Can you work these out from the drawing? Everything is in mm from the part's minimum corner. Give positions to 0.01 mm unless a question says otherwise; leave off trailing zeros. Order: outer loops, then holes, each group sorted by start corner. A loop starts at its lowest first (then second) coordinate and runs counter-clockwise, first axis right, second up. Notation, with made-up numbers: (9.25, 17.25) - (26.25, 17.25) arc R22 ccw to (26.25, 29.25) - close; hole circle Ø11 at (64.25, -18). An arc over 180 degrees is marked (long way). Answer as a JSON object with one key per item and string values.
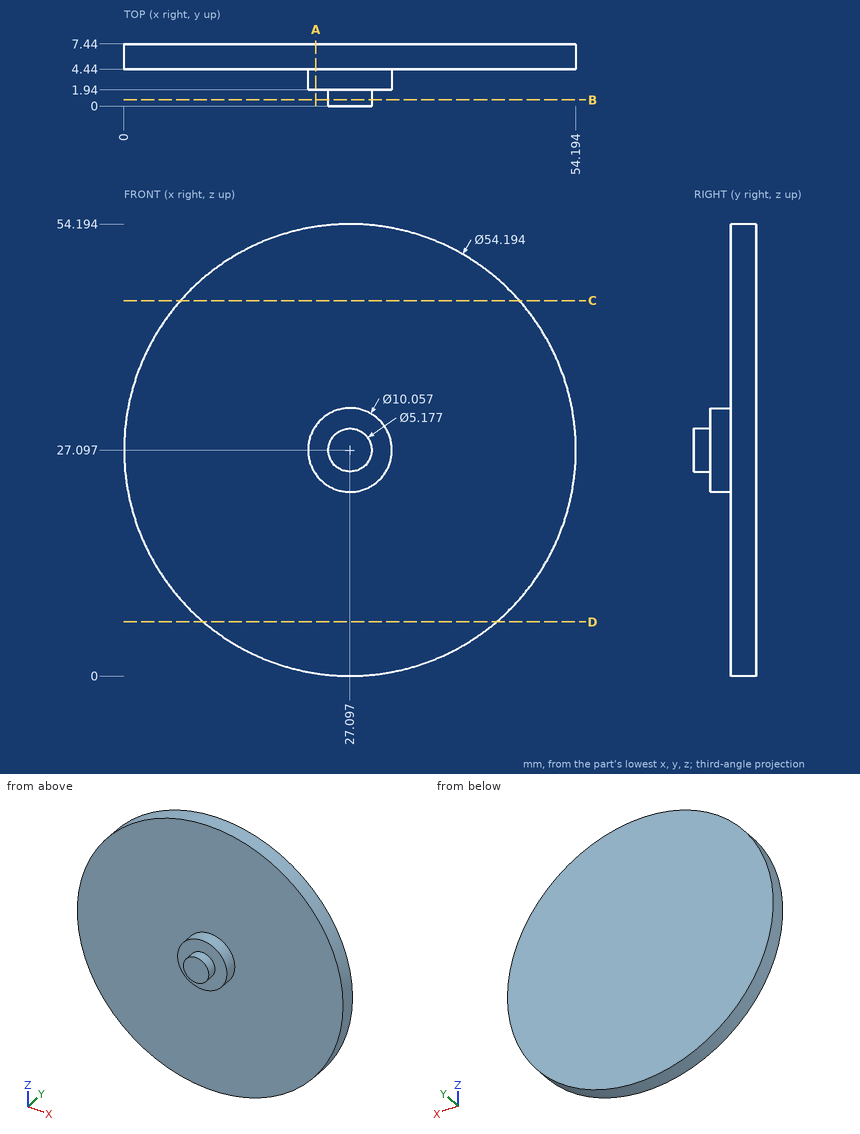
Q1. If we section it at B-B, the plane y = 0.75: Please give me the cut outline in (x, z) (1 decimal).
Recorded:
{"outline": "circle Ø5.2 at (27.1, 27.1)"}
Q2. If we section it at A-A, the plane x = 23: Please give me the cut outline in (y, z).
Recorded:
{"outline": "(1.94, 24.18) - (4.44, 24.18) - (4.44, 0.31) - (7.44, 0.31) - (7.44, 53.88) - (4.44, 53.88) - (4.44, 30.01) - (1.94, 30.01) - close"}
Q3. If we section it at D-D, the plane z = 6.5: Please give me the cut outline in (x, y), then the cut area to 3 significant figures.
Recorded:
{"outline": "(9.49, 4.44) - (44.7, 4.44) - (44.7, 7.44) - (9.49, 7.44) - close", "area": "106 mm^2"}
Q4. If we section it at C-C, the plane z = 45: Please give me the cut outline in (x, y).
Recorded:
{"outline": "(6.76, 4.44) - (47.44, 4.44) - (47.44, 7.44) - (6.76, 7.44) - close"}
Q5. I'm going to push flat-ended pins straight in: pin 1 Ø3 at (x, z) = (26.5, 24.5) entering from -Y; pin 2 Ø1.5 at (y, z) = (4.5, 33.5) entering from -X; pin 3 Ø1.5 at (y, z) = (4.5, 47) entering from -X; pin 4 Ø1.5 at (y, z) = (4, 30) entering from -X. Where does each tip first touch, or does it pass through?
Recorded:
{"pin 1": "stops at y = 0", "pin 2": "stops at x = 0.6", "pin 3": "stops at x = 7.93", "pin 4": "stops at x = 0.1"}
Q6. I need wall thicknesses on L1, parallel to Y at x = 23, z = 37.5; L2, parallel to Z at x = 43, y = 6.5 (1 decimal); L3, parallel to X at y = 5.25, z = 19.5. Which ranges of each line are inside material? Lowest first, please.
Recorded:
{"L1": "y = 4.44 to 7.44", "L2": "z = 5.2 to 49", "L3": "x = 1.09 to 53.11"}
